```python
from build123d import *

# Parameters (mm, degrees)
F0_R           = 50
F0_R_2         = 28.5
F1_DEPTH       = 47.5
F2_DEPTH       = 47.5
F3_D           = 6.8
F3_DEPTH       = 23.75
F3_CBORE_D     = 6.8
F3_CBORE_DEPTH = 1
F3_TIP         = 2.0429261047
F4_DEPTH       = 2.5


with BuildPart() as f1:
    # F0 (on Top) → F1 (new body)
    with BuildSketch(Plane.XY):
        Circle(F0_R)
        with BuildLine():
            ThreePointArc((37.7707857076, 17.193537944), (40.5569821786, 8.7966582614), (41.5, 0))
            ThreePointArc((41.5, 0), (40.5569821786, -8.7966582614), (37.7707857076, -17.193537944))
            ThreePointArc((37.7707857076, -17.193537944), (39.3549426741, -18.6670844715), (39.9400542571, -20.75))
            ThreePointArc((39.9400542571, -20.75), (37.8559766131, -24.2613019702), (33.7754334942, -24.1136909717))
            ThreePointArc((33.7754334942, -24.1136909717), (20.75, -35.9400542571), (3.9953522134, -41.3072289157))
            ThreePointArc((3.9953522134, -41.3072289157), (3.9988378845, -41.4035864469), (4, -41.5))
            ThreePointArc((4, -41.5), (-0.0964135531, -45.4988378845), (-3.9953522134, -41.3072289157))
            ThreePointArc((-3.9953522134, -41.3072289157), (-20.75, -35.9400542571), (-33.7754334942, -24.1136909717))
            ThreePointArc((-33.7754334942, -24.1136909717), (-39.4041558722, -22.75), (-37.7707857076, -17.193537944))
            ThreePointArc((-37.7707857076, -17.193537944), (-41.5, 0), (-37.7707857076, 17.193537944))
            ThreePointArc((-37.7707857076, 17.193537944), (-39.4041558722, 22.75), (-33.7754334942, 24.1136909717))
            ThreePointArc((-33.7754334942, 24.1136909717), (-20.75, 35.9400542571), (-3.9953522134, 41.3072289157))
            ThreePointArc((-3.9953522134, 41.3072289157), (-0.0964135531, 45.4988378845), (4, 41.5))
            ThreePointArc((4, 41.5), (3.9988378845, 41.4035864469), (3.9953522134, 41.3072289157))
            ThreePointArc((3.9953522134, 41.3072289157), (20.75, 35.9400542571), (33.7754334942, 24.1136909717))
            ThreePointArc((33.7754334942, 24.1136909717), (37.8559766131, 24.2613019702), (39.9400542571, 20.75))
            ThreePointArc((39.9400542571, 20.75), (39.3549426741, 18.6670844715), (37.7707857076, 17.193537944))
        make_face(mode=Mode.SUBTRACT)
        with BuildLine():
            ThreePointArc((37.7707857076, -17.193537944), (40.5569821786, -8.7966582614), (41.5, 0))
            ThreePointArc((41.5, 0), (40.5569821786, 8.7966582614), (37.7707857076, 17.193537944))
            ThreePointArc((37.7707857076, 17.193537944), (32.4759526419, 18.75), (33.7754334942, 24.1136909717))
            ThreePointArc((33.7754334942, 24.1136909717), (20.75, 35.9400542571), (3.9953522134, 41.3072289157))
            ThreePointArc((3.9953522134, 41.3072289157), (0, 37.5), (-3.9953522134, 41.3072289157))
            ThreePointArc((-3.9953522134, 41.3072289157), (-20.75, 35.9400542571), (-33.7754334942, 24.1136909717))
            ThreePointArc((-33.7754334942, 24.1136909717), (-32.4287522869, 22.665922356), (-31.9400542571, 20.75))
            ThreePointArc((-31.9400542571, 20.75), (-33.8571387285, 17.3351115829), (-37.7707857076, 17.193537944))
            ThreePointArc((-37.7707857076, 17.193537944), (-41.5, 0), (-37.7707857076, -17.193537944))
            ThreePointArc((-37.7707857076, -17.193537944), (-33.8571387285, -17.3351115829), (-31.9400542571, -20.75))
            ThreePointArc((-31.9400542571, -20.75), (-32.4287522869, -22.665922356), (-33.7754334942, -24.1136909717))
            ThreePointArc((-33.7754334942, -24.1136909717), (-20.75, -35.9400542571), (-3.9953522134, -41.3072289157))
            ThreePointArc((-3.9953522134, -41.3072289157), (0, -37.5), (3.9953522134, -41.3072289157))
            ThreePointArc((3.9953522134, -41.3072289157), (20.75, -35.9400542571), (33.7754334942, -24.1136909717))
            ThreePointArc((33.7754334942, -24.1136909717), (32.4759526419, -18.75), (37.7707857076, -17.193537944))
        make_face()
        Circle(F0_R_2, mode=Mode.SUBTRACT)
        with BuildLine():
            ThreePointArc((-37.7707857076, 17.193537944), (-35.9400542571, 20.75), (-33.7754334942, 24.1136909717))
            ThreePointArc((-33.7754334942, 24.1136909717), (-39.4041558722, 22.75), (-37.7707857076, 17.193537944))
        make_face()
        with BuildLine():
            ThreePointArc((-37.7707857076, -17.193537944), (-39.4041558722, -22.75), (-33.7754334942, -24.1136909717))
            ThreePointArc((-33.7754334942, -24.1136909717), (-35.9400542571, -20.75), (-37.7707857076, -17.193537944))
        make_face()
        with BuildLine():
            ThreePointArc((4, -41.5), (3.9988378845, -41.4035864469), (3.9953522134, -41.3072289157))
            ThreePointArc((3.9953522134, -41.3072289157), (0, -41.5), (-3.9953522134, -41.3072289157))
            ThreePointArc((-3.9953522134, -41.3072289157), (-0.0964135531, -45.4988378845), (4, -41.5))
        make_face()
        with BuildLine():
            ThreePointArc((39.9400542571, -20.75), (39.3549426741, -18.6670844715), (37.7707857076, -17.193537944))
            ThreePointArc((37.7707857076, -17.193537944), (35.9400542571, -20.75), (33.7754334942, -24.1136909717))
            ThreePointArc((33.7754334942, -24.1136909717), (37.8559766131, -24.2613019702), (39.9400542571, -20.75))
        make_face()
        with BuildLine():
            ThreePointArc((33.7754334942, 24.1136909717), (35.9400542571, 20.75), (37.7707857076, 17.193537944))
            ThreePointArc((37.7707857076, 17.193537944), (39.3549426741, 18.6670844715), (39.9400542571, 20.75))
            ThreePointArc((39.9400542571, 20.75), (37.8559766131, 24.2613019702), (33.7754334942, 24.1136909717))
        make_face()
        with BuildLine():
            ThreePointArc((-3.9953522134, 41.3072289157), (0, 41.5), (3.9953522134, 41.3072289157))
            ThreePointArc((3.9953522134, 41.3072289157), (3.9988378845, 41.4035864469), (4, 41.5))
            ThreePointArc((4, 41.5), (-0.0964135531, 45.4988378845), (-3.9953522134, 41.3072289157))
        make_face()
        with BuildLine():
            ThreePointArc((-31.9400542571, 20.75), (-32.4287522869, 22.665922356), (-33.7754334942, 24.1136909717))
            ThreePointArc((-33.7754334942, 24.1136909717), (-35.9400542571, 20.75), (-37.7707857076, 17.193537944))
            ThreePointArc((-37.7707857076, 17.193537944), (-33.8571387285, 17.3351115829), (-31.9400542571, 20.75))
        make_face()
        with BuildLine():
            ThreePointArc((-37.7707857076, -17.193537944), (-35.9400542571, -20.75), (-33.7754334942, -24.1136909717))
            ThreePointArc((-33.7754334942, -24.1136909717), (-32.4287522869, -22.665922356), (-31.9400542571, -20.75))
            ThreePointArc((-31.9400542571, -20.75), (-33.8571387285, -17.3351115829), (-37.7707857076, -17.193537944))
        make_face()
        with BuildLine():
            ThreePointArc((-3.9953522134, -41.3072289157), (0, -41.5), (3.9953522134, -41.3072289157))
            ThreePointArc((3.9953522134, -41.3072289157), (0, -37.5), (-3.9953522134, -41.3072289157))
        make_face()
        with BuildLine():
            ThreePointArc((33.7754334942, -24.1136909717), (35.9400542571, -20.75), (37.7707857076, -17.193537944))
            ThreePointArc((37.7707857076, -17.193537944), (32.4759526419, -18.75), (33.7754334942, -24.1136909717))
        make_face()
        with BuildLine():
            ThreePointArc((33.7754334942, 24.1136909717), (32.4759526419, 18.75), (37.7707857076, 17.193537944))
            ThreePointArc((37.7707857076, 17.193537944), (35.9400542571, 20.75), (33.7754334942, 24.1136909717))
        make_face()
        with BuildLine():
            ThreePointArc((-3.9953522134, 41.3072289157), (0, 37.5), (3.9953522134, 41.3072289157))
            ThreePointArc((3.9953522134, 41.3072289157), (0, 41.5), (-3.9953522134, 41.3072289157))
        make_face()
    extrude(amount=-F1_DEPTH)

    # F0 (on Top) → F2 (join)
    with BuildSketch(Plane.XY):
        Circle(F0_R_2)
        with BuildLine():
            ThreePointArc((5, 16.7705098312), (0, -17.5), (-5, 16.7705098312))
            Line((-5, 16.7705098312), (-5, 20.7705098312))
            Line((-5, 20.7705098312), (5, 20.7705098312))
            Line((5, 20.7705098312), (5, 16.7705098312))
        make_face(mode=Mode.SUBTRACT)
    extrude(amount=-F2_DEPTH)

    # F3
    with Locations(Plane.XY):
        with Locations((35.9400542571, -20.75), (35.9400542571, 20.75), (0, 41.5), (-35.9400542571, 20.75), (-35.9400542571, -20.75), (0, -41.5)):
            CounterBoreHole(F3_D / 2, F3_CBORE_D / 2, F3_CBORE_DEPTH, depth=F3_DEPTH)
            with Locations((0, 0, -(F3_DEPTH + F3_TIP / 2))):  # 118° drill point
                Cone(0, F3_D / 2, F3_TIP, mode=Mode.SUBTRACT)

    # F0 (on Top) → F4 (join)
    with BuildSketch(Plane.XY):
        Circle(F0_R_2)
        with BuildLine():
            ThreePointArc((5, 16.7705098312), (0, -17.5), (-5, 16.7705098312))
            Line((-5, 16.7705098312), (-5, 20.7705098312))
            Line((-5, 20.7705098312), (5, 20.7705098312))
            Line((5, 20.7705098312), (5, 16.7705098312))
        make_face(mode=Mode.SUBTRACT)
    extrude(amount=F4_DEPTH)


solid = f1.part
```
Design review of the part built by this model. Coordinates are the model's own, in mm. A direction names the side the tool comes from. Coordinates: 2 decimals unless noted, no trailing zeros. Order: outer loops, then holes, each group sorted by start corner. A loop starts at its lowest first (then second) coordinate and runs counter-clockwise, first axis right, second up. Notation, with made-up numbers: (47.5, 81) - (86.5, 81) arc R13 cw to (86.5, 106) - close; hole circle Ø6 at (20.25, 21). An arc over 180 degrees is marked (long way). Answer in a Markdown table with one row per item.
(1) Consider section A-A on z = -11.5. State the section outline as (x, y) points, plus the area to 3 significant figures.
Checked values:
| item | result |
|---|---|
| outline | circle Ø100 at (0, 0); hole circle Ø6.8 at (-35.94, -20.75); hole circle Ø6.8 at (-35.94, 20.75); hole (-5, 16.77) arc R17.5 ccw (long way) to (5, 16.77) - (5, 20.77) - (-5, 20.77) - close; hole circle Ø6.8 at (0, -41.5); hole circle Ø6.8 at (0, 41.5); hole circle Ø6.8 at (35.94, -20.75); hole circle Ø6.8 at (35.94, 20.75) |
| area | 6,640 mm^2 |
(2) Wall thickness on line 1 along Y through (x, z) = (0, -9); line 2 along Z through (x, y) = (-17, 40.5); line 3 along X through (y, z) = (-18, -21): over which ranges is each line inside the solid? List them lowest first. Write a range as from..to.
Checked values:
| item | result |
|---|---|
| line 1 | -50..-44.9, -38.1..-17.5, 20.77..38.1, 44.9..50 |
| line 2 | -47.5..0 |
| line 3 | -46.65..-37.94, -33.94..33.94, 37.94..46.65 |
(3) For faces 4 (the cylindrical face through (-39.08, -22.05, -12.04)), 5 (the flat face through (0, 20.771, -23)), 6 (the flat face through (-1, -22, -47.5)), list the 3-axis set-ups (+Z, -Z, +X, -X, +Y, -Y) from which the entire face can be reached by the end or side of a thin tool; tool diameter is ignored.
Checked values:
| item | result |
|---|---|
| face 4 | +Z |
| face 5 | +Z, -Z |
| face 6 | -Z, +X, -X, +Y, -Y |
(4) Clearance check with flat-ended pins moving along their axes: pin 1 (5 mm diameter, centred on x = 2.5, z = -23.5, fed in from -Y); pin 2 (2 mm diameter, centred on x = 37, y = -11.5, fed in from +Z); pin 3 (6 mm diameter, centred on y = 17.5, z = -19, fed in from +X). State where each tip first meets the part, or that it passes through.
Checked values:
| item | result |
|---|---|
| pin 1 | y = -50 |
| pin 2 | z = 0 |
| pin 3 | x = 47.85 |
(5) Consider section C-C on x = -13.5. State the section outline as (y, z) points, plus the area to 3 significant figures.
Checked values:
| item | result |
|---|---|
| outline | (-48.14, -47.5) - (-11.14, -47.5) - (-11.14, 2.5) - (-25.1, 2.5) - (-25.1, 0) - (-48.14, 0) - close; (11.14, -47.5) - (48.14, -47.5) - (48.14, 0) - (25.1, 0) - (25.1, 2.5) - (11.14, 2.5) - close |
| area | 3,590 mm^2 |
(6) The part is to be moulded in two halves that separate along Y. For faces 1 (the cylindrical face through (26.327, -10.916, 1.232)), 2 (the conical face through (36.257, 21.248, -25.438)), 3 (the flat face through (22, -22, 0)), say which applies: released by +Y, released by -Y, zero draft, split by the parting line, or undercut.
Checked values:
| item | result |
|---|---|
| face 1 | split by the parting line |
| face 2 | undercut |
| face 3 | zero draft |
(7) Consider section B-B on y = 0. State the section outline as (x, z) points, plus the area to 3 significant figures.
Checked values:
| item | result |
|---|---|
| outline | (-50, -47.5) - (-17.5, -47.5) - (-17.5, 2.5) - (-28.5, 2.5) - (-28.5, 0) - (-50, 0) - close; (17.5, -47.5) - (50, -47.5) - (50, 0) - (28.5, 0) - (28.5, 2.5) - (17.5, 2.5) - close |
| area | 3,140 mm^2 |
(8) Consider section D-D on z = -37.5. State the section outline as (x, y) points.
Checked values:
| item | result |
|---|---|
| outline | circle Ø100 at (0, 0); hole (-5, 16.77) arc R17.5 ccw (long way) to (5, 16.77) - (5, 20.77) - (-5, 20.77) - close |
